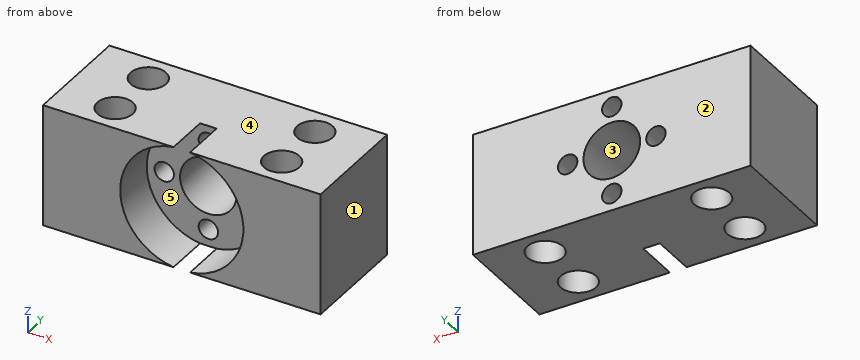
```python
from build123d import *

# Parameters (mm, degrees)
SKETCH_W        = 50
SKETCH_H        = 20
SKETCH_R        = 3.2
PAD_DEPTH       = 22
SKETCH001_R     = 11.1
POCKET_DEPTH    = 8
SKETCH002_R     = 5.1
SKETCH002_R_2   = 1.75
POCKET001_DEPTH = 20


with BuildPart() as part:
    # Sketch → Pad (new body)
    with BuildSketch(Plane.XY):
        with Locations((25, 10)):
            Rectangle(SKETCH_W, SKETCH_H)
        with Locations((10, 15)):
            Circle(SKETCH_R, mode=Mode.SUBTRACT)
        with Locations((10, 5)):
            Circle(SKETCH_R, mode=Mode.SUBTRACT)
        with Locations((40, 15)):
            Circle(SKETCH_R, mode=Mode.SUBTRACT)
        with Locations((40, 5)):
            Circle(SKETCH_R, mode=Mode.SUBTRACT)
    extrude(amount=PAD_DEPTH)

    # Sketch001 (on Face3 of Pad) → Pocket (cut)
    with BuildSketch(Plane.XZ):
        with Locations((25, 11)):
            Circle(SKETCH001_R)
    extrude(amount=-POCKET_DEPTH, mode=Mode.SUBTRACT)

    # Sketch002 (on Face1 of Pocket) → Pocket001 (cut)
    with BuildSketch(Plane(origin=(0, 20, 0), x_dir=(-1, 0, 0), z_dir=(0, 1, 0))):
        with Locations((-25, 11)):
            Circle(SKETCH002_R)
        with Locations((-25, 18.95)):
            Circle(SKETCH002_R_2)
        with Locations((-25, 3.05)):
            Circle(SKETCH002_R_2)
        with Locations((-32.95, 11)):
            Circle(SKETCH002_R_2)
        with Locations((-17.05, 11)):
            Circle(SKETCH002_R_2)
    extrude(amount=-POCKET001_DEPTH, mode=Mode.SUBTRACT)


solid = part.part
```
Check sheet for the modelled part. Datum: model origin and axes. Units: mm. Face numbers are marked on the shaded views. A direction names the side the tool comes from. Round coordinates to 2 decimals unless told otherwise and drop trailing zeros. Loops run counter-clockwise (first coordinate to the right, second up) from the corner with the lowest first, then second, coordinate; pieces in that order, holes last. Notation, with made-up numbers: (-29.5, 1) - (24.5, 1) arc R35 ccw to (24.5, 37) - close; hole circle Ø2 at (19, 8.25). An arc over 180 degrees is marked (long way). Answer as a JSON object with one key per item and string values. Group by question number.
Q1. Sectioned sample at A-A, the plane y = 15. Enter the section's corners in (x, z).
Q2. Set-up check for the marked faces 4 and 5: record each of +Z, -Z, +X, -X, +Y, -Y from which the full face is reachable in a straight line by a thin tool's end or side.
Q3. Sectioned sample at D-D, the plane x = 10. Enter the section's corners in (y, z), plus the area to 3 significant figures.
Q4. Gauge pin test, flat ends, axial feed: P1, Ø6, axis at x = 10, y = 5, coming from the +Z side; P2, Ø11.5, axis at x = 25, z = 11, coming from the -Y side. Record the tip position at first contact, or that the pin passes through.
Q5. Mould release check, pull along X, two halves, no side actions. Record for the marked faces 1, 2 and 3: released by +X, released by -X, zero draft, split by the parting line, or undercut.
Q6. Sectioned sample at B-B, the plane z = 11. Enter the section's corners in (x, y), plus the area to 3 significant figures.
Q7. Scan lines: line 1 along Y through (x, z) = (10, 9); line 2 along Z through (x, y) = (25, 16.5); line 3 along X through (y, z) = (12.5, 20). Record each from-to range of solid material in increasing order. Write a range as [from, to].
Q8. Sectioned sample at C-C, the plane z = 2.25. Enter the section's corners in (x, y), plus the area to 3 significant figures.
Solution:
{
 "1": {"outline": "(0, 0) - (6.8, 0) - (6.8, 22) - (0, 22) - close; (13.2, 0) - (36.8, 0) - (36.8, 22) - (13.2, 22) - close; (43.2, 0) - (50, 0) - (50, 22) - (43.2, 22) - close; hole circle Ø3.5 at (17.05, 11); hole circle Ø10.2 at (25, 11); hole circle Ø3.5 at (25, 3.05); hole circle Ø3.5 at (25, 18.95); hole circle Ø3.5 at (32.95, 11)"},
 "2": {"face 4": "+Z, +X, -X, +Y, -Y", "face 5": "-Y"},
 "3": {"outline": "(0, 0) - (1.8, 0) - (1.8, 22) - (0, 22) - close; (8.2, 0) - (11.8, 0) - (11.8, 22) - (8.2, 22) - close; (18.2, 0) - (20, 0) - (20, 22) - (18.2, 22) - close", "area": "158 mm²"},
 "4": {"P1": "passes through", "P2": "stops at y = 8"},
 "5": {"face 1": "released by +X", "face 2": "zero draft", "face 3": "undercut"},
 "6": {"outline": "(0, 0) - (13.9, 0) - (13.9, 8) - (15.3, 8) - (15.3, 20) - (0, 20) - close; (18.8, 8) - (19.9, 8) - (19.9, 20) - (18.8, 20) - close; (30.1, 8) - (31.2, 8) - (31.2, 20) - (30.1, 20) - close; (34.7, 8) - (36.1, 8) - (36.1, 0) - (50, 0) - (50, 20) - (34.7, 20) - close; hole circle Ø6.4 at (10, 5); hole circle Ø6.4 at (10, 15); hole circle Ø6.4 at (40, 5); hole circle Ø6.4 at (40, 15)", "area": "487 mm²"},
 "7": {"line 1": "y = [0, 1.8], [8.2, 11.8], [18.2, 20]", "line 2": "z = [0, 1.3], [4.8, 5.9], [16.1, 17.2], [20.7, 22]", "line 3": "x = [0, 8], [12, 23.6], [26.4, 38], [42, 50]"},
 "8": {"outline": "(0, 0) - (18.17, 0) - (18.17, 8) - (23.44, 8) - (23.44, 20) - (0, 20) - close; (26.56, 8) - (31.83, 8) - (31.83, 0) - (50, 0) - (50, 20) - (26.56, 20) - close; hole circle Ø6.4 at (10, 5); hole circle Ø6.4 at (10, 15); hole circle Ø6.4 at (40, 5); hole circle Ø6.4 at (40, 15)", "area": "725 mm²"}
}
